```python
from build123d import *

# Parameters (mm, degrees)
SKETCH_1_R          = 135
SKETCH_1_R_2        = 2
SKETCH_1_W          = 40
SKETCH_1_H          = 62
SKETCH_1_R_3        = 1.75
EXTRUDE_1_DEPTH     = 3
FILLET_1_R          = 5
SKETCH_2_R          = 20
SKETCH_2_R_2        = 2
SKETCH_2_R_3        = 1.6
CUT_EXTRUDE_1_DEPTH = 10


with BuildPart() as part:
    # 草图1 → 凸台-拉伸1 (new body)
    with BuildSketch(Plane.XY):
        Circle(SKETCH_1_R)
        with Locations((-14.4, -110.804246301)):
            Circle(SKETCH_1_R_2, mode=Mode.SUBTRACT)
        with Locations((-20, -99.304246301)):
            Circle(SKETCH_1_R_2, mode=Mode.SUBTRACT)
        with Locations((-14.4, -87.804246301)):
            Circle(SKETCH_1_R_2, mode=Mode.SUBTRACT)
        with Locations((14.4, -110.804246301)):
            Circle(SKETCH_1_R_2, mode=Mode.SUBTRACT)
        with Locations((14.4, -87.804246301)):
            Circle(SKETCH_1_R_2, mode=Mode.SUBTRACT)
        with Locations((20, -99.304246301)):
            Circle(SKETCH_1_R_2, mode=Mode.SUBTRACT)
        with Locations((-86, 49.65212315)):
            Rectangle(SKETCH_1_W, SKETCH_1_H, mode=Mode.SUBTRACT)
        with Locations((-53, 34.65212315)):
            Circle(SKETCH_1_R_3, mode=Mode.SUBTRACT)
        with Locations((-53, 64.65212315)):
            Circle(SKETCH_1_R_3, mode=Mode.SUBTRACT)
        with Locations((-29, 34.65212315)):
            Circle(SKETCH_1_R_3, mode=Mode.SUBTRACT)
        with Locations((-29, 64.65212315)):
            Circle(SKETCH_1_R_3, mode=Mode.SUBTRACT)
        with Locations((29, 34.65212315)):
            Circle(SKETCH_1_R_3, mode=Mode.SUBTRACT)
        with Locations((29, 64.65212315)):
            Circle(SKETCH_1_R_3, mode=Mode.SUBTRACT)
        with Locations((53, 34.65212315)):
            Circle(SKETCH_1_R_3, mode=Mode.SUBTRACT)
        with Locations((53, 64.65212315)):
            Circle(SKETCH_1_R_3, mode=Mode.SUBTRACT)
        with Locations((86, 49.65212315)):
            Rectangle(SKETCH_1_W, SKETCH_1_H, mode=Mode.SUBTRACT)
    extrude(amount=EXTRUDE_1_DEPTH)

    # 圆角1
    fillet_1_edges = [part.edges().sort_by_distance(p)[0] for p in [
        (66, 80.65212315, 1.5),
        (66, 18.65212315, 1.5),
        (106, 18.65212315, 1.5),
        (106, 80.65212315, 1.5),
        (-106, 80.65212315, 1.5),
        (-106, 18.65212315, 1.5),
        (-66, 18.65212315, 1.5),
        (-66, 80.65212315, 1.5),
    ]]
    fillet(fillet_1_edges, radius=FILLET_1_R)

    # 草图2 → 切除-拉伸1 (cut)
    with BuildSketch(Plane.XY.offset(3)):
        Circle(SKETCH_2_R)
        with Locations((-72, 97)):
            Circle(SKETCH_2_R_2)
        with Locations((72, 97)):
            Circle(SKETCH_2_R_2)
        with Locations((72, -97)):
            Circle(SKETCH_2_R_2)
        with Locations((-72, -97)):
            Circle(SKETCH_2_R_2)
        with Locations((-60, 94)):
            Circle(SKETCH_2_R_3)
        with Locations((-60, 14)):
            Circle(SKETCH_2_R_3)
        with Locations((-40, 94)):
            Circle(SKETCH_2_R_3)
        with Locations((-40, 14)):
            Circle(SKETCH_2_R_3)
        with Locations((60, 14)):
            Circle(SKETCH_2_R_3)
        with Locations((60, 94)):
            Circle(SKETCH_2_R_3)
        with Locations((40, 94)):
            Circle(SKETCH_2_R_3)
        with Locations((40, 14)):
            Circle(SKETCH_2_R_3)
        with Locations((-39, -15.5)):
            Circle(SKETCH_2_R_3)
        with Locations((19, -15.5)):
            Circle(SKETCH_2_R_3)
        with Locations((-39, -64.5)):
            Circle(SKETCH_2_R_3)
        with Locations((19, -64.5)):
            Circle(SKETCH_2_R_3)
        with BuildLine():
            Line((24.505636669, -55), (53, -55))
            ThreePointArc((53, -55), (56, -58), (53, -61))
            Line((53, -61), (24.505636669, -61))
            ThreePointArc((24.505636669, -61), (21.505636669, -58), (24.505636669, -55))
        make_face()
        with BuildLine():
            Line((-53, -19), (-24.505636669, -19))
            ThreePointArc((-24.505636669, -19), (-21.505636669, -22), (-24.505636669, -25))
            Line((-24.505636669, -25), (-53, -25))
            ThreePointArc((-53, -25), (-56, -22), (-53, -19))
        make_face()
        with BuildLine():
            Line((-53, -61), (-24.505636669, -61))
            ThreePointArc((-24.505636669, -61), (-21.505636669, -58), (-24.505636669, -55))
            Line((-24.505636669, -55), (-53, -55))
            ThreePointArc((-53, -55), (-56, -58), (-53, -61))
        make_face()
        with BuildLine():
            Line((24.505636669, -25), (53, -25))
            ThreePointArc((53, -25), (56, -22), (53, -19))
            Line((53, -19), (24.505636669, -19))
            ThreePointArc((24.505636669, -19), (21.505636669, -22), (24.505636669, -25))
        make_face()
        with BuildLine():
            Line((-70, -30), (-70, -50))
            ThreePointArc((-70, -50), (-65, -55), (-60, -50))
            Line((-60, -50), (-60, -30))
            ThreePointArc((-60, -30), (-65, -25), (-70, -30))
        make_face()
        with BuildLine():
            Line((60, -30), (60, -50))
            ThreePointArc((60, -50), (65, -55), (70, -50))
            Line((70, -50), (70, -30))
            ThreePointArc((70, -30), (65, -25), (60, -30))
        make_face()
        with BuildLine():
            Line((-36.755588957, 121.9), (36.755588957, 121.9))
            ThreePointArc((36.755588957, 121.9), (38.655588957, 120), (36.755588957, 118.1))
            Line((36.755588957, 118.1), (-36.755588957, 118.1))
            ThreePointArc((-36.755588957, 118.1), (-38.655588957, 120), (-36.755588957, 121.9))
        make_face()
        with BuildLine():
            Line((-36.755588957, -118.1), (36.755588957, -118.1))
            ThreePointArc((36.755588957, -118.1), (38.655588957, -120), (36.755588957, -121.9))
            Line((36.755588957, -121.9), (-36.755588957, -121.9))
            ThreePointArc((-36.755588957, -121.9), (-38.655588957, -120), (-36.755588957, -118.1))
        make_face()
        with BuildLine():
            Line((12.5, -70.7), (-12.5, -70.7))
            ThreePointArc((-12.5, -70.7), (-14.1, -69.1), (-12.5, -67.5))
            Line((-12.5, -67.5), (12.5, -67.5))
            ThreePointArc((12.5, -67.5), (14.1, -69.1), (12.5, -70.7))
        make_face()
        with BuildLine():
            Line((20, 101), (-20, 101))
            ThreePointArc((-20, 101), (-24, 97), (-20, 93))
            Line((-20, 93), (20, 93))
            ThreePointArc((20, 93), (24, 97), (20, 101))
        make_face()
    extrude(amount=-CUT_EXTRUDE_1_DEPTH, mode=Mode.SUBTRACT)


solid = part.part
```
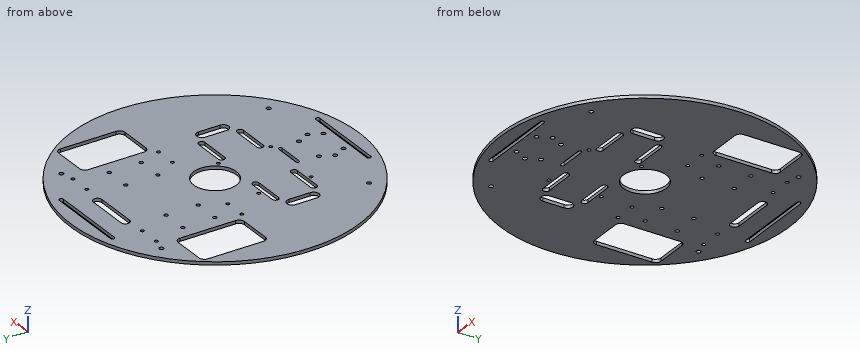
Could you check a few things on this model? Use its own coordinates, in mm. Round coordinates to 2 decimals unless told otherwise and drop trailing zeros. Loops run counter-clockwise (first coordinate to the right, second up) from the corner with the lowest first, then second, coordinate; pieces in that order, holes last. Notation, with made-up numbers: M -19.75,4 L 33.25,4 A33 ccw 33.25,33 Z; hole C -11.75,5 d9. An arc over 180 degrees is marked long. Put each result on its own line as item: value.
Q1. For pin 1 (1.5 mm diameter, centred on y = 68, z = 1, fed in from +X); pin 2 (1.5 mm diameter, centred on y = -44.5, z = 1, fed in from -X); pin 3 (3.5 mm diameter, centred on x = 72, y = 97, fed in from +Z); pin 4 (1 mm diameter, centred on y = -85, z = 2.5, fed in from +X), each with a flat end and sliding along its axis, tell me the tip position at first contact or that it passes through.
Check result:
pin 1: x = 117.06
pin 2: x = -127.71
pin 3: through
pin 4: x = 105.28
Q2. Imagine slicing it at A-A (x = 0). Write out the boundary of the cut face in (y, z), then the cut area to 3 significant figures.
Check result:
outline: M -135,0 L -121.9,0 L -121.9,3 L -135,3 Z; M -118.1,0 L -70.7,0 L -70.7,3 L -118.1,3 Z; M -67.5,0 L -20,0 L -20,3 L -67.5,3 Z; M 20,0 L 93,0 L 93,3 L 20,3 Z; M 101,0 L 118.1,0 L 118.1,3 L 101,3 Z; M 121.9,0 L 135,0 L 135,3 L 121.9,3 Z
area: 634 mm2
Q3. Imagine slicing it at C-C (z = 1.8). State how many separate pieces and enclosed holes the cut face has, then the cut area to 3 significant figures.
Check result:
separate pieces: 1
enclosed holes: 43
area: 48,400 mm2
Q4. Imagine slicing it at D-D (x = 118.5). Write out the boundary of the cut face in (y, z).
Check result:
outline: M -64.67,0 L 64.67,0 L 64.67,3 L -64.67,3 Z
Q5. Imagine slicing it at B-B (x = 84.5). Write out the boundary of the cut face in (y, z), then the cut area to 3 significant figures.
Check result:
outline: M -105.28,0 L 18.65,0 L 18.65,3 L -105.28,3 Z; M 80.65,0 L 105.28,0 L 105.28,3 L 80.65,3 Z
area: 446 mm2
Q6. I need wall thicknesses on probe 1 along X at (y, z) = (68.5, 0.85); probe 2 along Y at (x, z) = (40, 1.6); probe 3 along X at (y, z) = (-57, 2.6). Which ranges of each line are inside material? Lowest first, please.
Check result:
probe 1: -116.33 to -106, -66 to 66, 106 to 116.33
probe 2: -128.94 to -61, -55 to -25, -19 to 12.4, 15.6 to 92.4, 95.6 to 128.94
probe 3: -122.38 to -55.83, -21.68 to 21.68, 55.83 to 122.38
